from build123d import *

# Parameters (mm, degrees)
BOSS_EXTRUDE1_DEPTH = 9
SKETCH2_R           = 2.75
CUT_EXTRUDE1_DEPTH  = 21
SKETCH3_R           = 2.75
CUT_EXTRUDE2_DEPTH  = 21


with BuildPart() as part:
    # Sketch1 → Boss-Extrude1 (new body, symmetric)
    with BuildSketch(Plane.XY):
        with BuildLine():
            Line((0, 0), (0, 20))
            ThreePointArc((0, 20), (2.121320344, 19.121320344), (3, 17))
            Line((3, 17), (3, 6))
            ThreePointArc((3, 6), (3.878679656, 3.878679656), (6, 3))
            Line((6, 3), (17, 3))
            ThreePointArc((17, 3), (19.121320344, 2.121320344), (20, 0))
            Line((20, 0), (0, 0))
        make_face()
    extrude(amount=BOSS_EXTRUDE1_DEPTH, both=True)

    # Sketch2 → Cut-Extrude1 (cut, through all)
    with BuildSketch(Plane(origin=(0, 0, 0), x_dir=(1, 0, 0), z_dir=(0, 1, 0))):
        with Locations((10, 0)):
            Circle(SKETCH2_R)
    extrude(amount=CUT_EXTRUDE1_DEPTH, mode=Mode.SUBTRACT)

    # Sketch3 → Cut-Extrude2 (cut, through all)
    with BuildSketch(Plane(origin=(0, 0, 0), x_dir=(0, 0, -1), z_dir=(1, 0, 0))):
        with Locations((0, 10)):
            Circle(SKETCH3_R)
    extrude(amount=CUT_EXTRUDE2_DEPTH, mode=Mode.SUBTRACT)


solid = part.part
Verification items for the finished model (mm, model axes). A direction names the side the tool comes from. Give positions to 0.01 mm unless a question says otherwise; leave off trailing zeros. Write each loop counter-clockwise with the first axis right and the second up, starting at its lowest first coordinate (ties: lowest second). Pieces come first, ordered by that corner, then holes. Notation, with made-up numbers: M -6,62.5 L 0,62.5 A16 ccw 0,68.5 Z; hole C -14,-39.75 d9. An arc over 180 degrees is marked long. Write item = value, one per line.
(1) Go/stop test with flat-tipped pins: pin 1 Ø2 at (y, z) = (2.5, -4.5) entering from +X; pin 2 Ø3.5 at (y, z) = (11, 2) entering from +X; pin 3 Ø4 at (x, z) = (16, -7) entering from +Y; pin 4 Ø12 at (x, y) = (12, 17) entering from -Z. Record where each tip stops, or that it passes through.
Found:
pin_1 = 19.6
pin_2 = 3
pin_3 = 3
pin_4 = through
(2) Sectioned sample at D-D (z = 7). Record the cut outline in (x, y), then the cut area to 3 significant figures.
Found:
outline = M 0,0 L 20,0 A3 ccw 17,3 L 6,3 A3 cw 3,6 L 3,17 A3 ccw 0,20 Z
area = 109 mm2
(3) Draft check along X on faces 1 (the face through (3, 13, 0)), 2 (the face through (12.4, 0, -1.9)), 3 (the face through (12.54, 1.48, 1.05)). Enter one of: released by +X, released by -X, zero draft, split by the parting line, or undercut.
Found:
face_1 = released by +X
face_2 = zero draft
face_3 = undercut
(4) Sectioned sample at B-B (z = 0). Record the cut outline in (x, y).
Found:
outline = M 0,0 L 7.25,0 L 7.25,3 L 6,3 A3 cw 3,6 L 3,7.25 L 0,7.25 Z; M 0,12.75 L 3,12.75 L 3,17 A3 ccw 0,20 Z; M 12.75,0 L 20,0 A3 ccw 17,3 L 12.75,3 Z
(5) Material ranges on line 1 (Z direction, x = 10, y = 0.6); line 2 (Y direction, x = 10.5, z = -6.5), recorded low to high.
Found:
line_1 = -9 to -2.75, 2.75 to 9
line_2 = 0 to 3
(6) Access from +Z, -Z, +X, -X, +Y, -Y to the whole of each face (thin tool, end or side, straight path). Record for faces 4 (the face through (4, 3, -9)), 5 (the face through (13, 3, 2)).
Found:
face_4 = -Z, +X, -X, +Y, -Y
face_5 = +Z, -Z, +X, +Y
(7) Sectioned sample at A-A (y = 10). Record the cut outline in (x, z), then the cut area to 3 significant figures.
Found:
outline = M 0,-9 L 3,-9 L 3,-2.75 L 0,-2.75 Z; M 0,2.75 L 3,2.75 L 3,9 L 0,9 Z
area = 37.5 mm2
